Verification items for the finished model (mm, model axes). A direction names the side the tool comes from. Give positions to 0.01 mm unless a question says otherwise; leave off trailing zeros. Write each loop counter-clockwise with the first axis right and the second up, starting at its lowest first coordinate (ties: lowest second). Pieces come first, ordered by that corner, then holes. Notation, with made-up numbers: (-22.75, 49.25) -> (18.25, 49.25) arc R12 cw to (18.25, 67.25) -> close; hole circle Ø7 at (32, -17). An arc over 180 degrees is marked (long way). Answer as CSV lines item,"result".
```python
from build123d import *

# Parameters (mm, degrees)
SKETCH1_R           = 0.79375
BOSS_EXTRUDE1_DEPTH = 2.794
FILLET1_R           = 6.35
FILLET2_R           = 3.175


with BuildPart() as part:
    # Sketch1 → Boss-Extrude1 (new body)
    with BuildSketch(Plane.XY):
        with BuildLine():
            Line((-15.237072382, 13.269795383), (-8.887072382, 13.269795383))
            Line((-8.887072382, 13.269795383), (-8.887072382, -5.780204617))
            Line((-8.887072382, -5.780204617), (-6.220072382, -5.780204617))
            Line((-6.220072382, -5.780204617), (-6.220072382, 32.313013632))
            Line((-6.220072382, 32.313013632), (-6.220072382, 76.769795383))
            Line((-6.220072382, 76.769795383), (19.179927297, 76.769795383))
            ThreePointArc((19.179927297, 76.769795383), (31.879927297, 64.069795092), (19.179926715, 51.369795383))
            ThreePointArc((19.179926715, 51.369795383), (9.654926277, 41.844795383), (19.179926715, 32.319795383))
            ThreePointArc((19.179926715, 32.319795383), (38.229927618, 13.269795835), (19.179927618, -5.780204617))
            Line((19.179927618, -5.780204617), (19.179927618, -18.480204617))
            Line((19.179927618, -18.480204617), (-15.237072382, -18.480204617))
            Line((-15.237072382, -18.480204617), (-15.237072382, 13.269795383))
        make_face()
        with Locations((19.179927618, 13.269795383)):
            Circle(SKETCH1_R, mode=Mode.SUBTRACT)
        with Locations((19.179927618, 64.069795383)):
            Circle(SKETCH1_R, mode=Mode.SUBTRACT)
    extrude(amount=BOSS_EXTRUDE1_DEPTH)

    # Fillet1
    fillet1_edges = [part.edges().sort_by_distance(p)[0] for p in [
        (19.179927618, -18.480204617, 1.397),
        (-6.220072382, 76.769795383, 1.397),
    ]]
    fillet(fillet1_edges, radius=FILLET1_R)

    # Fillet2
    fillet2_edges = [part.edges().sort_by_distance(p)[0] for p in [
        (-15.237072382, -18.480204617, 1.397),
    ]]
    fillet(fillet2_edges, radius=FILLET2_R)


solid = part.part
```
1) Section check A-A (x = 15.5). Record the boundary of the cut face in (y, z), and give its area (3 significant figures).
Reported:
outline,"(-17.89, 0) -> (33.06, 0) -> (33.06, 2.79) -> (-17.89, 2.79) -> close; (50.63, 0) -> (76.77, 0) -> (76.77, 2.79) -> (50.63, 2.79) -> close"
area,"215 mm²"
2) Scan lines: line 1 along Y through (x, z) = (26, 1.25); line 2 along X through (y, z) = (-6, 2.5); line 3 along Y through (x, z) = (25.5, 0.5). Record each from-to range of solid material in increasing order.
Reported:
line 1,"-4.52 to 31.06, 53.36 to 74.78"
line 2,"-15.24 to 19.18"
line 3,"-4.7 to 31.24, 53.05 to 75.09"
3) Section check B-B (y = 1). Record the boundary of the cut face in (x, z).
Reported:
outline,"(-15.24, 0) -> (-8.89, 0) -> (-8.89, 2.79) -> (-15.24, 2.79) -> close; (-6.22, 0) -> (33.75, 0) -> (33.75, 2.79) -> (-6.22, 2.79) -> close"
4) Draft check along Y on faces 1 (the flat face through (10, 76.77, 1)), 2 (the cylindrical face through (31.877, 64.349, 1.377)), 3 (the flat face through (-8.887, 4, 1)). Enter one of: +Y half, -Y half, draft (parallel to the pull), parting line (faces both ways), or undercut.
Reported:
face 1,"+Y half"
face 2,"undercut"
face 3,"draft"
5) Tool access check on faces 4 (the flat face through (12, 30, 0)), 5 (the flat face through (19.18, -9, 1)), 6 (the flat face through (-8, -5.78, 1)), 7 (the flat face through (-12, 13.27, 1)), 8 (the flat face through (-15.237, -1, 1)). Record the directions out of +Z, -Z, +X, -X, +Y, -Y that give a thin tool (end or side, any length) a straight path to the whole face; none if there is none.
Reported:
face 4,"-Z, +X, -X, +Y, -Y"
face 5,"+Z, -Z, +X, -Y"
face 6,"+Z, -Z, +Y"
face 7,"+Z, -Z, -X, +Y"
face 8,"+Z, -Z, -X, +Y, -Y"
6) Section check C-C (z = 1.9). State how many separate pieces and enclosed holes the cut face has, and give its area (3 significant figures).
Reported:
separate pieces,"1"
enclosed holes,"2"
area,"3,310 mm²"
7) Depth check by flat-ended pin: pin 1 (1.8 mm diameter, centred on x = 19.18, y = 64.07, fed in from +Z); pin 2 (1.3 mm diameter, centred on x = -7.5, z = 1.5, fed in from +Y); pin 3 (0.8 mm diameter, centred on y = -9.5, z = 1, fed in from +X). Enter the tip coordinate at first touch or a pass-through.
Reported:
pin 1,"z = 2.79"
pin 2,"y = -5.78"
pin 3,"x = 19.18"
8) Section check D-D (y = -10.5). Record the boundary of the cut face in (x, z), and give its area (3 significant figures).
Reported:
outline,"(-15.24, 0) -> (19.18, 0) -> (19.18, 2.79) -> (-15.24, 2.79) -> close"
area,"96.2 mm²"
